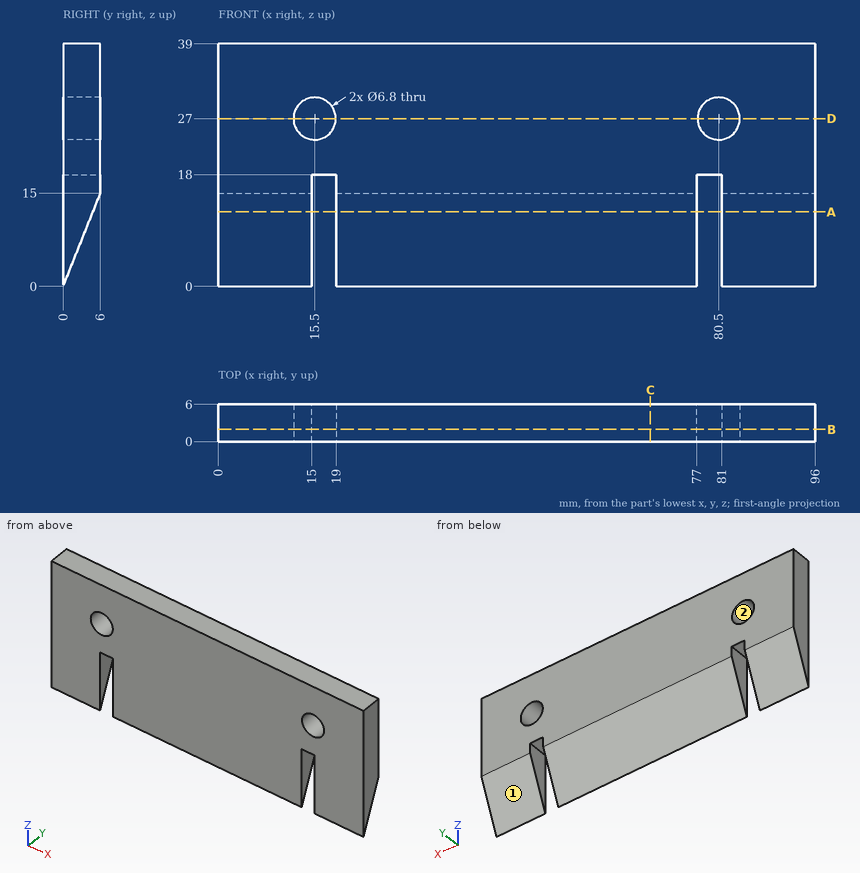
Verification items for this drawing (mm, ordinates from the low corner). Coordinates: 2 decimals unless noted, no trailing zeros. Write each loop counter-clockwise with the first axis right and the second up, starting at its lowest first coordinate (ties: lowest second). Pieces come first, ordered by that corner, then holes. Notation, with made-up numbers: (-13.5, 81) -> (34.5, 81) arc R28 cw to (34.5, 113) -> close; hole circle Ø1 at (16, 78.5). An arc over 180 degrees is marked (long way). Use CSV: the item, a comma, the result in double quotes. Start each with the question number.
Item 1: Cross-section at D-D, the plane z = 27. Record the cut outline in (x, y).
Item 2: Cross-section at B-B, the plane y = 2. Record the cut outline in (x, z).
Item 3: Depth check by flat-ended pin: pin 1 Ø3 at (y, z) = (4, 9) entering from -X; pin 2 Ø1.2 at (x, y) = (78.5, 3) entering from -Z; pin 3 Ø1 at (x, y) = (32, 4) entering from -Z. Enter the tip coordinate at first touch or a pass-through.
Item 4: Mould release check, pull along X, two halves, no side actions. Record for the marked faces 1 and 2: released by +X, released by -X, zero draft, split by the parting line, or undercut.
Item 5: Cross-section at C-C, the plane x = 69.5. Record the cut outline in (y, z).
Item 6: Thickness scan on line 1 (X direction, y = 2.6, z = 27); line 2 (Z direction, x = 80.5, y = 1.65); line 3 (Z direction, x = 78, y = 4). Record the ranges inside material, lowest first.
Item 7: Cross-section at A-A, the plane z = 12. Record the cut outline in (x, y).
Answers:
1,outline,"(0, 0) -> (12.1, 0) -> (12.1, 6) -> (0, 6) -> close; (18.9, 0) -> (77.1, 0) -> (77.1, 6) -> (18.9, 6) -> close; (83.9, 0) -> (96, 0) -> (96, 6) -> (83.9, 6) -> close"
2,outline,"(0, 5) -> (15, 5) -> (15, 18) -> (19, 18) -> (19, 5) -> (77, 5) -> (77, 18) -> (81, 18) -> (81, 5) -> (96, 5) -> (96, 39) -> (0, 39) -> close; hole circle Ø6.8 at (15.5, 27); hole circle Ø6.8 at (80.5, 27)"
3,pin 1,"x = 0"
3,pin 2,"z = 18"
3,pin 3,"z = 8.75"
4,face 1,"zero draft"
4,face 2,"undercut"
5,outline,"(0, 0) -> (6, 15) -> (6, 39) -> (0, 39) -> close"
6,line 1,"0 to 12.1, 18.9 to 77.1, 83.9 to 96"
6,line 2,"18 to 23.6, 30.4 to 39"
6,line 3,"18 to 24.7, 29.3 to 39"
7,outline,"(0, 0) -> (15, 0) -> (15, 4.8) -> (0, 4.8) -> close; (19, 0) -> (77, 0) -> (77, 4.8) -> (19, 4.8) -> close; (81, 0) -> (96, 0) -> (96, 4.8) -> (81, 4.8) -> close"
